Can you work these out from the model? Positions are in its coordinate system, mm. A direction names the side the tool comes from. Coordinates: 2 decimals unless noted, no trailing zeros. Write each question's results on one line, items separated by ' | '. Start each with the question number.
```python
from build123d import *

# Parameters (mm, degrees)
BOSS_EXTRU_1_DEPTH             = 150
FRACTIONNER1_SURFACE_1_BACK    = 338.186
FRACTIONNER1_SURFACE_1_DEPTH   = 676.372
FRACTIONNER1_SURFACE_2_BACK    = 338.186
FRACTIONNER1_SURFACE_2_DEPTH   = 676.372
CORPS_SUPPRIMER_GARDER_1_DEPTH = 150
ESQUISSE4_W                    = 70
ESQUISSE4_H                    = 27
ENL_V_MAT_EXTRU_1_DEPTH        = 20


with BuildPart() as part:
    # Esquisse1 → Boss.-Extru.1 (new body)
    with BuildSketch(Plane.XY):
        with BuildLine():
            ThreePointArc((300, 0.615), (300.57616321, 0), (300, -0.615))
            add(Edge.make_bspline(
                [(300, 0.615), (297.904984084, 0.751757543), (292.317834147, 1.116473101), (283.239167486, 1.717548993), (272.763851073, 2.401734129), (262.289009769, 3.093148372), (251.814135815, 3.784066551), (241.337843931, 4.4686253), (230.862161266, 5.161453759), (220.385838201, 5.845538162), (209.911154414, 6.538349242), (199.435845553, 7.222650253), (188.961161962, 7.915464365), (178.484838114, 8.599536639), (168.010154067, 9.292344726), (157.534847028, 9.976669832), (147.06015641, 10.669390538), (136.583858848, 11.353812357), (126.108081003, 12.045381523), (115.628989204, 12.734847578), (106.544413863, 13.318771764), (98.151476207, 13.759261663), (91.156562369, 14.075053545), (83.459091103, 14.332671008), (76.809762769, 14.494266326), (71.208103955, 14.553043896), (68.057010771, 14.564841535), (65.955984612, 14.566136146), (63.504942858, 14.548307662), (58.950185243, 14.50722741), (52.639372933, 14.342178025), (45.976395003, 14.041169691), (40.714278866, 13.694270896), (36.853148612, 13.371585869), (33.690528003, 13.066756335), (30.525686443, 12.713592883), (27.357424626, 12.304603807), (23.829347777, 11.773145061), (20.293449043, 11.155810812), (16.752613493, 10.405038809), (13.91014568, 9.695268378), (11.411898729, 8.968942676), (9.247069544, 8.239122328), (7.047101664, 7.371563533), (5.204368253, 6.469298236), (3.704406867, 5.566960218), (2.492406306, 4.671764118), (0.823776108, 3.084389444), (-0.563560511, 0), (0.823776108, -3.084389444), (2.492406306, -4.671764118), (3.704406867, -5.566960218), (5.204368253, -6.469298236), (7.047101664, -7.371563533), (9.247069544, -8.239122328), (11.411898729, -8.968942676), (13.91014568, -9.695268378), (16.752613493, -10.405038809), (20.293449043, -11.155810812), (23.829347777, -11.773145061), (27.357424626, -12.304603807), (30.525686443, -12.713592883), (33.690528003, -13.066756335), (36.853148612, -13.371585869), (40.714278866, -13.694270896), (45.976395003, -14.041169691), (52.639372933, -14.342178025), (58.950185243, -14.50722741), (63.504942858, -14.548307662), (65.955984612, -14.566136146), (68.057010771, -14.564841535), (71.208103955, -14.553043896), (76.809762769, -14.494266326), (83.459091103, -14.332671008), (91.156562369, -14.075053545), (98.151476207, -13.759261663), (106.544413863, -13.318771764), (115.628989204, -12.734847578), (126.108081003, -12.045381523), (136.583858848, -11.353812357), (147.06015641, -10.669390538), (157.534847028, -9.976669832), (168.010154067, -9.292344726), (178.484838114, -8.599536639), (188.961161962, -7.915464365), (199.435845553, -7.222650253), (209.911154414, -6.538349242), (220.385838201, -5.845538162), (230.862161266, -5.161453759), (241.337843931, -4.4686253), (251.814135815, -3.784066551), (262.289009769, -3.093148372), (272.763851073, -2.401734129), (283.239167486, -1.717548993), (292.317834147, -1.116473101), (297.904984084, -0.751757543), (300, -0.615)],
                knots=[0, 0, 0, 0, 0.010331767, 0.027553552, 0.044775014, 0.061991889, 0.079213674, 0.096435137, 0.113656922, 0.130878384, 0.14810017, 0.165316721, 0.182538507, 0.199759969, 0.216981754, 0.234198306, 0.251420091, 0.268641554, 0.285863339, 0.303084802, 0.320322147, 0.330661097, 0.344443905, 0.354779244, 0.368562092, 0.377174559, 0.382346694, 0.384069086, 0.387513926, 0.39440881, 0.406484298, 0.418578438, 0.427229264, 0.432434172, 0.437645264, 0.442864528, 0.448104782, 0.453364927, 0.460421621, 0.465764879, 0.471174038, 0.474835156, 0.478565394, 0.482412615, 0.486466494, 0.488643966, 0.491021881, 0.493857902, 0.5, 0.506142098, 0.508978119, 0.511356034, 0.513533506, 0.517587385, 0.521434606, 0.525164844, 0.528825962, 0.534235121, 0.539578379, 0.546635073, 0.551895218, 0.557135472, 0.562354736, 0.567565828, 0.572770736, 0.581421562, 0.593515702, 0.60559119, 0.612486074, 0.615930914, 0.617653306, 0.622825441, 0.631437908, 0.645220756, 0.655556095, 0.669338903, 0.679677853, 0.696915198, 0.714136661, 0.731358446, 0.748579909, 0.765801694, 0.783018246, 0.800240031, 0.817461493, 0.834683279, 0.85189983, 0.869121616, 0.886343078, 0.903564863, 0.920786326, 0.938008111, 0.955224986, 0.972446448, 0.989668233, 1, 1, 1, 1], degree=3))
        make_face()
    extrude(amount=BOSS_EXTRU_1_DEPTH)


with BuildPart() as body_2:
    # Fractionner1: the piece behind the surface
    add(part.part)
    # Fractionner1 surface: a surface, the sketch's curves swept straight by 676.372 mm
    with BuildLine(Plane.XY.offset(150).offset(-FRACTIONNER1_SURFACE_1_BACK), mode=Mode.PRIVATE) as fractionner1_surface_1_path:
        Line((57.022091302, 21.120873497), (57.022091302, -26.585419846))
    fractionner1_surface_1 = Shell.extrude(fractionner1_surface_1_path.wire(), (0 * FRACTIONNER1_SURFACE_1_DEPTH, 0 * FRACTIONNER1_SURFACE_1_DEPTH, 1 * FRACTIONNER1_SURFACE_1_DEPTH))
    split(bisect_by=fractionner1_surface_1, keep=Keep.BOTTOM)

    # Corps-Supprimer/Garder 1: read off the stored shape, not the designer's step
    # Corps-Supprimer/Garder 1 outline → Corps-Supprimer/Garder 1 (cut)
    with BuildSketch(Plane.XY):
        with BuildLine():
            Line((57.022091311, -14.449616285), (57.022091311, 14.449616285))
            add(Edge.make_bspline(
                [(57.022091311, 14.449616285), (55.562497262, 14.414805897), (51.646493469, 14.297323458), (45.976395003, 14.041169691), (40.714278866, 13.694270896), (36.853148612, 13.371585869), (33.690528003, 13.066756335), (30.525686443, 12.713592883), (27.357424626, 12.304603807), (23.829347777, 11.773145061), (20.293449043, 11.155810812), (16.752613493, 10.405038809), (13.91014568, 9.695268378), (11.411898729, 8.968942676), (9.247069544, 8.239122328), (7.047101664, 7.371563533), (5.204368253, 6.469298236), (3.704406867, 5.566960218), (2.492406306, 4.671764118), (0.823776108, 3.084389444), (-0.563560511, 0), (0.823776108, -3.084389444), (2.492406306, -4.671764118), (3.704406867, -5.566960218), (5.204368253, -6.469298236), (7.047101664, -7.371563533), (9.247069544, -8.239122328), (11.411898729, -8.968942676), (13.91014568, -9.695268378), (16.752613493, -10.405038809), (20.293449043, -11.155810812), (23.829347777, -11.773145061), (27.357424626, -12.304603807), (30.525686443, -12.713592883), (33.690528003, -13.066756335), (36.853148612, -13.371585869), (40.714278866, -13.694270896), (45.976395003, -14.041169691), (51.646493469, -14.297323458), (55.562497262, -14.414805897), (57.022091311, -14.449616285)],
                knots=[0.399299529, 0.399299529, 0.399299529, 0.399299529, 0.406484298, 0.418578438, 0.427229264, 0.432434172, 0.437645264, 0.442864528, 0.448104782, 0.453364927, 0.460421621, 0.465764879, 0.471174038, 0.474835156, 0.478565394, 0.482412615, 0.486466494, 0.488643966, 0.491021881, 0.493857902, 0.5, 0.506142098, 0.508978119, 0.511356034, 0.513533506, 0.517587385, 0.521434606, 0.525164844, 0.528825962, 0.534235121, 0.539578379, 0.546635073, 0.551895218, 0.557135472, 0.562354736, 0.567565828, 0.572770736, 0.581421562, 0.593515702, 0.600700471, 0.600700471, 0.600700471, 0.600700471], degree=3))
        make_face()
    extrude(amount=CORPS_SUPPRIMER_GARDER_1_DEPTH, mode=Mode.SUBTRACT)


with BuildPart() as part_1:
    add(part.part)

    # Fractionner1: split by a surface, the side it looks to stays
    # Fractionner1 surface: a surface, the sketch's curves swept straight by 676.372 mm
    with BuildLine(Plane.XY.offset(150).offset(-FRACTIONNER1_SURFACE_2_BACK), mode=Mode.PRIVATE) as fractionner1_surface_2_path:
        Line((57.022091302, 21.120873497), (57.022091302, -26.585419846))
    fractionner1_surface_2 = Shell.extrude(fractionner1_surface_2_path.wire(), (0 * FRACTIONNER1_SURFACE_2_DEPTH, 0 * FRACTIONNER1_SURFACE_2_DEPTH, 1 * FRACTIONNER1_SURFACE_2_DEPTH))
    split(bisect_by=fractionner1_surface_2, keep=Keep.TOP)

    # Esquisse4 → Enlèv. mat.-Extru.1 (cut)
    with BuildSketch(Plane.ZY.offset(-57.022091302)):
        with Locations((75, 0.035962925)):
            Rectangle(ESQUISSE4_W, ESQUISSE4_H)
    extrude(amount=-ENL_V_MAT_EXTRU_1_DEPTH, mode=Mode.SUBTRACT)


solid = part_1.part
```
Q1. Thinking about a two-plate mould opening in Y: for faces 3 (the face through (67, -13.464, 75)), 4 (the face through (77.022, 0, 75)), 5 (the face through (153, 0, 150)), which applies, pulls with the +Y half, pulls with the -Y half, needs draft (parallel to the pull), parting line crosses it, or undercut?
Q2. I need wall thicknesses on line 1 along Y through (x, z) = (73.5, 83); line 2 along Y through (x, z) = (92, 138.5); line 3 along Y through (x, z) = (189, 128). Which ranges of each line are inside material? Lowest first, please. Write a range as from..to.
Q3. I'm going to push flat-ended pins straight in: pin 1 Ø8 at (x, z) = (159, 65) entering from +Y; pin 2 Ø6 at (y, z) = (-6.5, 44) entering from -X; pin 3 Ø5 at (x, z) = (137.5, 47) entering from -Y. Where does each tip first touch, or does it pass through?
Q4. For faces 1 (the face through (67, 13.536, 75)), 2 (the face through (57.022, 0, 24)), which set-ups out of +Z, -Z, +X, -X, +Y, -Y let a thin tool reach every point of the face, with its end or its side?
Answer list:
1) face 3: undercut | face 4: undercut | face 5: needs draft
2) line 1: y = -14.53..-13.46, 13.54..14.53 | line 2: y = -14.03..14.03 | line 3: y = -7.91..7.91
3) pin 1: stops at y = 10.14 | pin 2: stops at x = 77.02 | pin 3: stops at y = -11.46
4) face 1: -X | face 2: +Z, -Z, -X, +Y, -Y
